Can you work these out from the model? Positions are in its coordinate system, mm. A direction names the side the tool comes from. Coordinates: 2 decimals unless noted, no trailing zeros. Order: outer loops, then holes, each group sorted by start corner. A loop starts at its lowest first (then second) coordinate and runs counter-clockwise, first axis right, second up. Notation, with made-up numbers: (78, 36) - (116, 36) arc R20 cw to (116, 47) - close; hole circle Ø11 at (87.25, 68.25). An arc over 180 degrees is marked (long way). Return JSON: item names as keys, results as strings. Group by question number.
1) Which directions (+Z, -Z, +X, -X, +Y, -Y) give clear straight access to the entire face, cutting with the end or side of a thin tool? Please do faces 5 (the face through (-1.154, 1, 0)), 6 (the face through (0.193, -3.535, -3.384)), 7 (the face through (-0.51, -8.46, -1.52)), 8 (the face through (1, -3, 3.554)), 9 (the face through (-3.154, -3.8, 0)).
2) Imagine slicing it at C-C (z = -0.25). Write out the boundary of the cut face in (x, y).
3) Imagine slicing it at B-B (y = -6.45). Write out the boundary of the cut face in (x, z).
4) Imagine slicing it at A-A (x = -1.5). Write out the boundary of the cut face in (y, z).
5) Imagine slicing it at D-D (x = 2.25). Write out the boundary of the cut face in (y, z), and give its area (3 significant figures).
6) For pin 1 Ø1 at (x, z) = (2, 2) entering from -Y; pin 2 Ø1.1 at (x, z) = (4.5, -0.5) entering from +Y; pin 3 Ø2 at (x, y) = (0, -1) entering from -Z; pin 4 Ø3.5 at (y, z) = (-6, -0.5) entering from -X, each with a flat end and sliding along its axis, tell me the tip position at first contact or that it passes through.
7) If I drill on line 1 along Y through (x, z) = (-2.2, 0); line 2 along Z through (x, y) = (-2.8, 1.55); line 3 along X through (y, z) = (-4.25, 3), over which ranges is the centre line in solid material (lowest first)?
8) If we mould it in two halves opening along Y, with no side actions, what happens to faces 1 (the face through (1.26, 3.31, 0.13)), 2 (the face through (1, -7.45, 0)), 3 (the face through (4.676, -8, 0)), 4 (the face through (3.303, -4, 0))? For each: pulls with the +Y half, pulls with the -Y half, needs draft (parallel to the pull), parting line crosses it, or undercut.
Autodesk Inventor part; units mm, degrees
ref_plane "YZ Plane" through (0, 0, 0) normal (1, 0, 0) x (0, 1, 0)
ref_plane "XZ Plane" through (0, 0, 0) normal (0, 1, 0) x (-1, 0, 0)
ref_plane "XY Plane" through (0, 0, 0) normal (0, 0, 1) x (1, 0, 0)
sketch "Sketch1" plane through (0, 0, 0) normal (0, 0, 1) x (1, 0, 0)
  line L0 (-3.154, -9.45) -> (4.676, -9.45)
  line L1 (4.676, -9.45) -> (4.676, -6.279)
  line L2 (4.676, -6.279) -> (3.303, -6.279)
  line L3 (3.303, -6.279) -> (3.303, -1.2735)
  line L4 (-3.154, -9.45) -> (-3.154, -1.6074)
  arc A0 (3.303, -1.2735) -> (-3.154, -1.6074) centre (0, 0) ccw
  dimension "d0" = 7.83
  dimension "d1" = 9.45
  dimension "d2" = 3.54
  dimension "d3" = 3.154
  dimension "d4" = 3.171
  dimension "d5" = 6.457
extrude "Extrusion1" add sketch "Sketch1" along normal mid plane 7.108
sketch "Sketch2" plane through (-3.154, -9.45, 3.554) normal (0, -1, 0) x (1, 0, 0)
  line L0 (7.83, -7.108) -> (7.83, 0)
  circle A0 centre (4.63, -3.554) radius 2.5
  point P0 (3.154, -3.554)
  dimension "d8" = 5
  dimension "d9" = 3.2
extrude "Extrusion2" cut sketch "Sketch2" against normal blind 2
sketch "Sketch3" plane through (-3.154, -9.45, 3.554) normal (-1, 0, 0) x (0, 0, 1)
  line L0 (0, 0) -> (-7.108, 0)
  circle A0 centre (-3.554, 3) radius 2.5
  point P0 (-3.554, 9.45)
  dimension "d12" = 5
  dimension "d13" = 3
extrude "Extrusion3" cut sketch "Sketch3" against normal blind 2
sketch "Sketch4" plane through (-1.154, -6.45, 0) normal (-1, 0, 0) x (0, 0, 1)
  circle A0 centre (0, 0) radius 2.5 construction
  circle A1 centre (0, 8) radius 2.5
  circle A2 centre (0, 0) radius 2.5
  point P0 (0, 6.45)
  dimension "d16" = 8
extrude "Extrusion4" cut sketch "Sketch4" along normal through all contours A1
sketch "Sketch5" plane through (0, 0, -3.554) normal (0, 0, -1) x (-1, 0, 0)
  arc A0 (3.154, -1.6074) -> (-3.303, -1.2735) centre (0, 0) ccw
  circle A1 centre (0, 0) radius 3.54
extrude "Extrusion5" cut sketch "Sketch5" against normal blind 0.345
fillet "Fillet1" radius 0.1 2 edges at (3.303, -1.2735, -3.3815) (-3.154, -1.6074, -3.3815)
properties part number "LEG LHS" material "250"
Calculated:
{
 "1": {"face 5": "-X", "face 6": "-Z, +Y", "face 7": "-Y", "face 8": "+Z, +X, -X, +Y, -Y", "face 9": "+Z, -Z, -X, -Y"},
 "2": {"outline": "(-3.41, -0.94) arc R3.54 ccw to (-3.15, -1.61) - (-3.15, -3.96) - (-1.15, -3.96) - (-1.15, -8.94) - (-3.15, -8.94) - (-3.15, -9.45) - (-1.01, -9.45) - (-1.01, -7.45) - (3.96, -7.45) - (3.96, -9.45) - (4.68, -9.45) - (4.68, -6.28) - (3.3, -6.28) - (3.3, -1.27) arc R3.54 ccw to (-1.15, 3.35) - (-1.15, -0.94) - close"},
 "3": {"outline": "(-3.15, -3.55) - (4.68, -3.55) - (4.68, 3.55) - (-3.15, 3.55) - (-3.15, 2.5) - (-1.15, 2.5) - (-1.15, -2.5) - (-3.15, -2.5) - close"},
 "4": {"outline": "(-9.45, -3.55) - (-3.21, -3.55) - (-3.21, -3.21) - (3.21, -3.21) - (3.21, -1.87) arc R2.5 cw (long way) to (3.21, 1.87) - (3.21, 3.55) - (-9.45, 3.55) - close; hole circle Ø5 at (-6.45, 0)"},
 "5": {"outline": "(-9.45, -3.55) - (-2.73, -3.55) - (-2.73, -3.21) - (2.73, -3.21) - (2.73, 3.55) - (-9.45, 3.55) - (-9.45, 2.38) - (-7.45, 2.38) - (-7.45, -2.38) - (-9.45, -2.38) - close", "area": "75.2 mm2"},
 "6": {"pin 1": "y = -9.45", "pin 2": "y = -6.28", "pin 3": "z = -3.21", "pin 4": "x = -1.15"},
 "7": {"line 1": "-9.45 to -8.95, -3.95 to -0.95", "line 2": "-3.21 to -2.5, 2.5 to 3.55", "line 3": "-3.15 to 3.3"},
 "8": {"face 1": "undercut", "face 2": "pulls with the -Y half", "face 3": "needs draft", "face 4": "undercut"}
}
